Geometry: final body of the model. Coordinates: model frame, mm. Coordinates: 2 decimals unless noted, no trailing zeros. Write each loop counter-clockwise with the first axis right and the second up, starting at its lowest first coordinate (ties: lowest second). Pieces come first, ordered by that corner, then holes. Notation, with made-up numbers: (24.5, 18) -> (63.5, 18) arc R30 cw to (63.5, 40) -> close; hole circle Ø9 at (36.25, 47.5). An arc over 180 degrees is marked (long way). One line per item, written item: value.
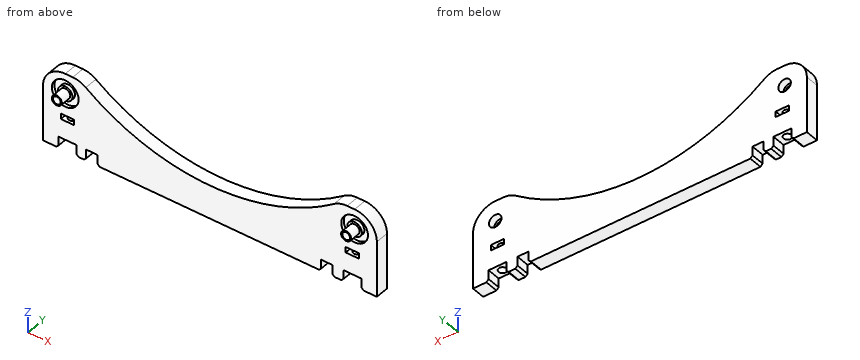
```python
from build123d import *

# Parameters (mm, degrees)
F1_DEPTH  = 6
F2_R      = 6
F2_R_2    = 3.25
F3_DEPTH  = 1.5
F4_W      = 8
F4_H      = 5
F4_W_2    = 6
F4_H_2    = 2.5
F4_W_3    = 5
F5_DEPTH  = 6.001
F6_R      = 10
F7_SIZE   = 1
F8_R      = 1.75
F9_DEPTH  = 14.5
F10_R     = 1.75
F11_DEPTH = 14.5
F12_R     = 2.25
F13_DEPTH = 5
F14_R     = 1.7
F15_DEPTH = 11.001
F16_R     = 2.25
F17_DEPTH = 5
F18_R     = 1.7
F19_DEPTH = 11.001
F20_R     = 2.8
F20_R_2   = 1.7
F21_DEPTH = 3


with BuildPart() as f1:
    # F0 (on Front) → F1 (new body)
    with BuildSketch(Plane.XZ):
        with BuildLine():
            Line((-75, 0), (75, 0))
            Line((75, 0), (75, 35))
            Line((75, 35), (58.3095189485, 35))
            ThreePointArc((58.3095189485, 35), (0, 15), (-58.3095189485, 35))
            Line((-58.3095189485, 35), (-75, 35))
            Line((-75, 35), (-75, 0))
        make_face()
    extrude(amount=F1_DEPTH)

    # F2 (on face) → F3 (cut)
    with BuildSketch(Plane.XZ.offset(6)):
        with Locations((-65, 26)):
            Circle(F2_R)
        with Locations((-65, 26)):
            Circle(F2_R_2, mode=Mode.SUBTRACT)
        with Locations((65, 26)):
            Circle(F2_R)
        with Locations((65, 26)):
            Circle(F2_R_2, mode=Mode.SUBTRACT)
    extrude(amount=-F3_DEPTH, mode=Mode.SUBTRACT)

    # F4 (on face) → F5 (cut, through all)
    with BuildSketch(Plane.XZ.offset(6)):
        with Locations((-64, 2.5)):
            Rectangle(F4_W, F4_H)
        with Locations((64, 2.5)):
            Rectangle(F4_W, F4_H)
        with Locations((-64, 14.75)):
            Rectangle(F4_W_2, F4_H_2)
        with Locations((64, 14.75)):
            Rectangle(F4_W_2, F4_H_2)
        with Locations((52.5, 2.5)):
            Rectangle(F4_W_3, F4_H)
        with Locations((-53.0885396898, 2.5)):
            Rectangle(F4_W_3, F4_H)
    extrude(amount=-F5_DEPTH, mode=Mode.SUBTRACT)

    # F6
    f6_edges = [f1.edges().sort_by_distance(p)[0] for p in [
        (-75, -3, 35),
        (75, -3, 35),
        (58.309519, -3, 35),
        (-58.309519, -3, 35),
    ]]
    fillet(f6_edges, radius=F6_R)

    # F7
    f7_edges = [f1.edges().sort_by_distance(p)[0] for p in [
        (-68, -3, 0),
        (-60, -3, 0),
        (60, -3, 0),
        (68, -3, 0),
        (-55.58854, -3, 0),
        (-50.58854, -3, 0),
        (50, -3, 0),
        (55, -3, 0),
    ]]
    chamfer(f7_edges, length=F7_SIZE)

    # F8 (on face) → F9 (cut)
    with BuildSketch(Plane(origin=(0, 0, 5), x_dir=(1, 0, 0), z_dir=(0, 0, -1))):
        with Locations((-64, 3)):
            Circle(F8_R)
    extrude(amount=-F9_DEPTH, mode=Mode.SUBTRACT)

    # F10 (on face) → F11 (cut)
    with BuildSketch(Plane(origin=(0, 0, 5), x_dir=(1, 0, 0), z_dir=(0, 0, -1))):
        with Locations((64, 3)):
            Circle(F10_R)
    extrude(amount=-F11_DEPTH, mode=Mode.SUBTRACT)

    # F12 (on face) → F13 (join)
    with BuildSketch(Plane.XZ.offset(6)):
        with Locations((-65, 26)):
            Circle(F12_R)
    extrude(amount=F13_DEPTH)

    # F14 (on face) → F15 (cut, through all)
    with BuildSketch(Plane.XZ.offset(11)):
        with Locations((-65, 26)):
            Circle(F14_R)
    extrude(amount=-F15_DEPTH, mode=Mode.SUBTRACT)

    # F16 (on face) → F17 (join)
    with BuildSketch(Plane.XZ.offset(6)):
        with Locations((65, 26)):
            Circle(F16_R)
    extrude(amount=F17_DEPTH)

    # F18 (on face) → F19 (cut, through all)
    with BuildSketch(Plane.XZ.offset(11)):
        with Locations((65, 26)):
            Circle(F18_R)
    extrude(amount=-F19_DEPTH, mode=Mode.SUBTRACT)

    # F20 (on face) → F21 (cut)
    with BuildSketch(Plane(origin=(0, 0, 0), x_dir=(-1, 0, 0), z_dir=(0, 1, 0))):
        with Locations((-65, 26)):
            Circle(F20_R)
        with Locations((-65, 26)):
            Circle(F20_R_2, mode=Mode.SUBTRACT)
        with Locations((65, 26)):
            Circle(F20_R)
        with Locations((65, 26)):
            Circle(F20_R_2, mode=Mode.SUBTRACT)
    extrude(amount=-F21_DEPTH, mode=Mode.SUBTRACT)


solid = f1.part
```
(1) Section B-B (x = 45.5). Return the cut outline in (y, z).
Responses:
outline: (-6, 0) -> (0, 0) -> (0, 26.6) -> (-6, 26.6) -> close
(2) Section C-C (x = 22). Return the cut outline in (y, z), then the cut area to 3 significant figures.
Responses:
outline: (-6, 0) -> (0, 0) -> (0, 17.58) -> (-6, 17.58) -> close
area: 105 mm2
(3) Line query: line 1 (X direction, y = -5.75, z = 4); line 2 (Y direction, x = 64, z = 18); line 3 (Z direction, x = 65, y = -1.8). Output: solid intervals per line, ascending. Write a range as [from, to].
Responses:
line 1: x = [-75, -68], [-60, -55.59], [-50.59, 50], [55, 60], [68, 75]
line 2: y = [-6, -4.75], [-1.25, 0]
line 3: z = [19.5, 23.2], [28.8, 35]
(4) Section A-A (z = 11.5). Return the cut outline in (x, y), then the cut area to 3 significant figures.
Responses:
outline: (-75, -6) -> (75, -6) -> (75, 0) -> (-75, 0) -> close; hole circle Ø3.5 at (-64, -3); hole circle Ø3.5 at (64, -3)
area: 881 mm2
(5) First-contact query: pin 1 (5.5 mm diameter, centred on x = -65, z = 26, fed in from -Y); pin 2 (4 mm diameter, centred on x = -52.5, y = -1.5, fed in from -Z); pin 3 (1.7 mm diameter, centred on x = -66, z = 25, fed in from +Y); pin 4 (10 mm diameter, centred on x = -5.5, z = 10.5, fed in from -Y). Flat tips, straight axial feed; report the tip coordinate or a pass-through.
Responses:
pin 1: stops at y = -11
pin 2: stops at z = 0.91
pin 3: stops at y = -3
pin 4: stops at y = -6
